The figure shows three views and two pictorial views of one solid part (mm, origin at its lowest corner). Answer the questions. Coordinates: 2 decimals unless noted, no trailing zeros. Order: outer loops, then holes, each group sorted by start corner. A loop starts at its lowest first (then second) coordinate and runs counter-clockwise, first axis right, second up. Notation, with made-up numbers: M 68,43.25 L 77,43.25 A18 cw 77,51.25 Z; hole C -25.75,43 d7. An arc over 180 degrees is marked long. Answer in a Markdown table with one row per item. Add a question column.
Item 1: The part is cut by section C-C (y = 20). Write down the section's boundary in (x, z).
Item 2: The part is cut by section A-A (z = 2.65). Write down the section's boundary in (x, y), then the cut area to 3 significant figures.
Item 3: The mould has two halves that part along Y. Classify the marked faces 1, 2, 3 and 4: released by +Y, released by -Y, zero draft, split by the parting line, or undercut.
Item 4: The part is cut by section D-D (y = 37). Write down the section's boundary in (x, z), then the cut area to 3 significant figures.
Item 5: Consider line 1 (Y direction, x = 10, z = 2.1); line 2 (X direction, y = 5, z = 1); line 3 (X direction, y = 6, z = 2.4). Determine where each line is inside the solid, lowest interval first. Write a range as from..to.
Item 6: The part is cut by section B-B (x = 10). Write down the section's boundary in (y, z).
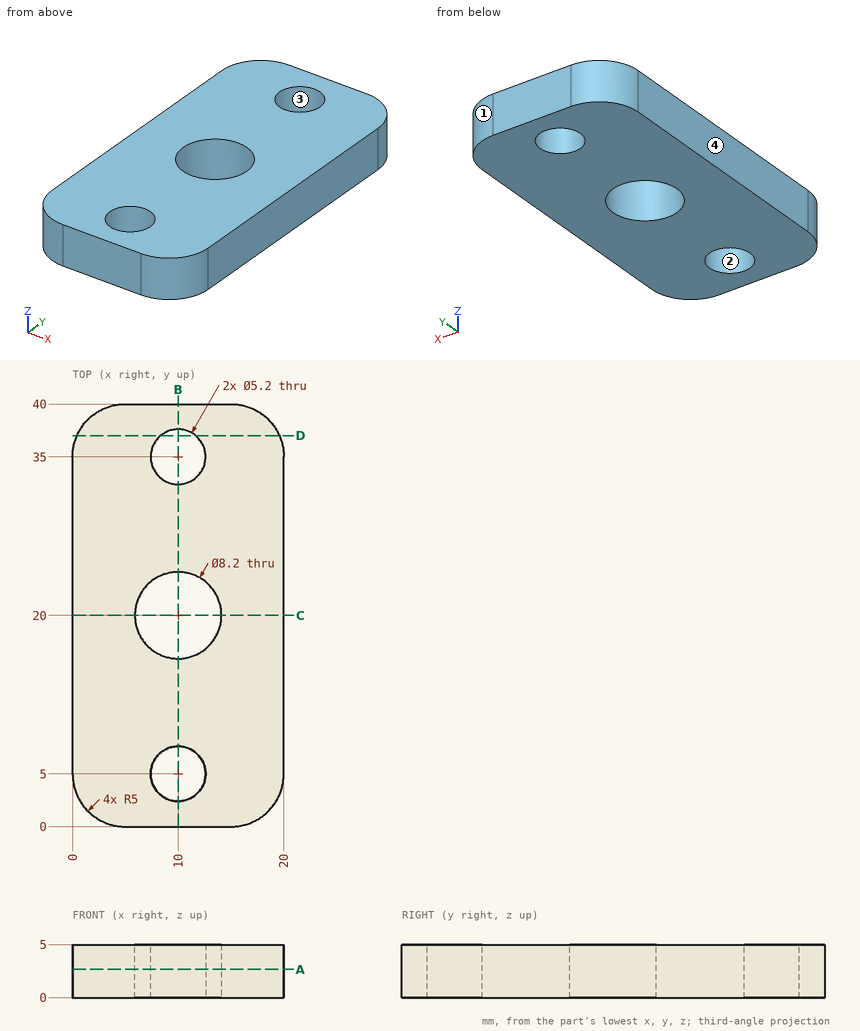
Reply:
| question | item | result |
|---|---|---|
| 1 | outline | M 0,0 L 5.9,0 L 5.9,5 L 0,5 Z; M 14.1,0 L 20,0 L 20,5 L 14.1,5 Z |
| 2 | outline | M 0,5 A5 ccw 5,0 L 15,0 A5 ccw 20,5 L 20,35 A5 ccw 15,40 L 5,40 A5 ccw 0,35 Z; hole C 10,20 d8.2; hole C 10,5 d5.2; hole C 10,35 d5.2 |
| 2 | area | 683 mm2 |
| 3 | face 1 | released by +Y |
| 3 | face 2 | undercut |
| 3 | face 3 | undercut |
| 3 | face 4 | zero draft |
| 4 | outline | M 0.42,0 L 8.34,0 L 8.34,5 L 0.42,5 Z; M 11.66,0 L 19.58,0 L 19.58,5 L 11.66,5 Z |
| 4 | area | 79.2 mm2 |
| 5 | line 1 | y = 0..2.4, 7.6..15.9, 24.1..32.4, 37.6..40 |
| 5 | line 2 | x = 0..7.4, 12.6..20 |
| 5 | line 3 | x = 0..7.6, 12.4..20 |
| 6 | outline | M 0,0 L 2.4,0 L 2.4,5 L 0,5 Z; M 7.6,0 L 15.9,0 L 15.9,5 L 7.6,5 Z; M 24.1,0 L 32.4,0 L 32.4,5 L 24.1,5 Z; M 37.6,0 L 40,0 L 40,5 L 37.6,5 Z |
